from build123d import *

# Parameters (mm, degrees)
F0_R     = 1.5
F1_DEPTH = 3
F2_W     = 3
F2_H     = 24
F3_DEPTH = 30
F4_R     = 1.5
F5_DEPTH = 25


with BuildPart() as f1:
    # F0 (on Top) → F1 (new body)
    with BuildSketch(Plane.XY):
        Polygon((-14, 0), (0, 0), (17, 0), (17, 24), (0, 24), (-14, 24), align=None)
        with Locations((0, 12)):
            Circle(F0_R, mode=Mode.SUBTRACT)
    extrude(amount=F1_DEPTH)

    # F2 (on face) → F3 (join)
    with BuildSketch(Plane.XY.offset(3)):
        with Locations((15.5, 12)):
            Rectangle(F2_W, F2_H)
    extrude(amount=F3_DEPTH)

    # F4 (on face) → F5 (cut)
    with BuildSketch(Plane.YZ.offset(17)):
        with Locations((6, 16)):
            Circle(F4_R)
        with Locations((18, 16)):
            Circle(F4_R)
    extrude(amount=-F5_DEPTH, mode=Mode.SUBTRACT)


solid = f1.part
Check sheet for the modelled part. Datum: model origin and axes. Units: mm. A direction names the side the tool comes from. Coordinates: 2 decimals unless noted, no trailing zeros. Loops run counter-clockwise (first coordinate to the right, second up) from the corner with the lowest first, then second, coordinate; pieces in that order, holes last. Notation, with made-up numbers: (19.25, 84) -> (31.25, 84) arc R16 cw to (31.25, 111) -> close; hole circle Ø3 at (89, 52). An arc over 180 degrees is marked (long way). Answer in a Markdown table with one row per item.
1. Sectioned sample at C-C, the plane z = 16. Record the boundary of the cut face in (x, y).
Check values:
| item | result |
|---|---|
| outline | (14, 0) -> (17, 0) -> (17, 4.5) -> (14, 4.5) -> close; (14, 7.5) -> (17, 7.5) -> (17, 16.5) -> (14, 16.5) -> close; (14, 19.5) -> (17, 19.5) -> (17, 24) -> (14, 24) -> close |
2. Sectioned sample at D-D, the plane z = 29.5. Record the boundary of the cut face in (x, y).
Check values:
| item | result |
|---|---|
| outline | (14, 0) -> (17, 0) -> (17, 24) -> (14, 24) -> close |
3. Go/stop test with flat-tipped pins: pin 1 (4 mm diameter, centred on y = 18, z = 16, fed in from -X); pin 2 (12 mm diameter, centred on x = 0, y = 14.5, fed in from +Z). Record where each tip stops, or that it passes through.
Check values:
| item | result |
|---|---|
| pin 1 | stops at x = 14 |
| pin 2 | stops at z = 3 |
4. Sectioned sample at B-B, the plane x = 0. Record the boundary of the cut face in (y, z), then the cut area to 3 significant figures.
Check values:
| item | result |
|---|---|
| outline | (0, 0) -> (10.5, 0) -> (10.5, 3) -> (0, 3) -> close; (13.5, 0) -> (24, 0) -> (24, 3) -> (13.5, 3) -> close |
| area | 63.0 mm2 |
5. Material ranges on line 1 along Y through (x, z) = (0, 1.4); line 2 along Z through (x, y) = (14.8, 6); line 3 along Z through (x, y) = (-11, 12.5), recorded low to high. Write a range as [from, to].
Check values:
| item | result |
|---|---|
| line 1 | y = [0, 10.5], [13.5, 24] |
| line 2 | z = [0, 14.5], [17.5, 33] |
| line 3 | z = [0, 3] |
6. Sectioned sample at A-A, the plane y = 18. Record the boundary of the cut face in (x, z), then the cut area to 3 significant figures.
Check values:
| item | result |
|---|---|
| outline | (-14, 0) -> (17, 0) -> (17, 14.5) -> (14, 14.5) -> (14, 3) -> (-14, 3) -> close; (14, 17.5) -> (17, 17.5) -> (17, 33) -> (14, 33) -> close |
| area | 174 mm2 |
7. Release check for a two-part mould opening along Z. For faces 1 (the face through (17, 12, 16)), 2 (the face through (1, 15, 0)), 3 (the face through (15.52, 16.5, 16.07)) record: released by +Z, released by -Z, zero draft, split by the parting line, or undercut.
Check values:
| item | result |
|---|---|
| face 1 | zero draft |
| face 2 | released by -Z |
| face 3 | undercut |
8. Access from +Z, -Z, +X, -X, +Y, -Y to the whole of each face (thin tool, end or side, straight path). Record for faces 4 (the face through (0, 15, 3)), 5 (the face through (-0.325, 10.536, 1.479)).
Check values:
| item | result |
|---|---|
| face 4 | +Z, -X, +Y, -Y |
| face 5 | +Z, -Z |
